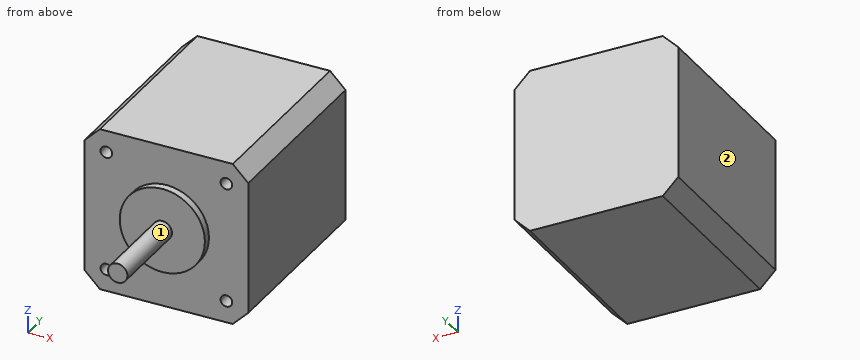
from build123d import *

# Parameters (mm, degrees)
F1_DEPTH = 48
F2_R     = 11
F3_DEPTH = 2
F4_R     = 2.5
F5_DEPTH = 22
F6_R     = 1.5
F7_DEPTH = 10


with BuildPart() as f1:
    # F0 (on Front) → F1 (new body)
    with BuildSketch(Plane.XZ):
        Polygon((17.15, 21.15), (0, 21.15), (-17.15, 21.15), (-21.15, 17.15), (-21.15, 0), (-21.15, -17.15), (-17.15, -21.15), (0, -21.15), (17.15, -21.15), (21.15, -17.15), (21.15, 0), (21.15, 17.15), align=None)
    extrude(amount=F1_DEPTH)

    # F2 (on face) → F3 (join)
    with BuildSketch(Plane.XZ.offset(48)):
        Circle(F2_R)
    extrude(amount=F3_DEPTH)

    # F4 (on face) → F5 (join)
    with BuildSketch(Plane.XZ.offset(50)):
        Circle(F4_R)
    extrude(amount=F5_DEPTH)

    # F6 (on face) → F7 (cut)
    with BuildSketch(Plane.XZ.offset(48)):
        with Locations((-15.5, 15.5)):
            Circle(F6_R)
        with Locations((15.5, 15.5)):
            Circle(F6_R)
        with Locations((-15.5, -15.5)):
            Circle(F6_R)
        with Locations((15.5, -15.5)):
            Circle(F6_R)
    extrude(amount=-F7_DEPTH, mode=Mode.SUBTRACT)


solid = f1.part
Geometry: final body of the model. Coordinates: model frame, mm. Face numbers are marked on the shaded views. A direction names the side the tool comes from. Give positions to 0.01 mm unless a question says otherwise; leave off trailing zeros. Write each loop counter-clockwise with the first axis right and the second up, starting at its lowest first coordinate (ties: lowest second). Pieces come first, ordered by that corner, then holes. Notation, with made-up numbers: M 26,30.5 L 85,30.5 A17 ccw 85,60.5 Z; hole C 73,23.5 d9. An arc over 180 degrees is marked long. Answer in a Markdown table with one row per item. Add a question column.
(1) Section C-C on z = 0. Return loops of the section in (x, y).
(2) Ray query, line 1 (Z direction, x = 15.5, y = -43.75); line 2 (Z direction, x = -15, y = -45); line 3 (Y direction, x = 0, z = 19.5). Return the intervals inside material, ascending.
(3) First-contact query: pin 1 (0.9 mm diameter, centred on x = 15, z = 15, fed in from -Y); pin 2 (4 mm diameter, centred on x = 15.5, z = 13, fed in from -Y); pin 3 (4 mm diameter, centred on x = 5.5, y = -52.5, fed in from +Z) (3 decimals). Flat tips, straight axial feed; report the tip coordinate or a pass-through.
(4) Section B-B on y = -17. Return loops of the section in (x, z), and give its area (3 significant figures).
(5) Section D-D on z = -6.5. Return loops of the section in (x, y).
(6) Reachability of the marked faces 1 and 2 from +Z, -Z, +X, -X, +Y, -Y: full face, straight path, thin tool, end or side. Return the list, or none.
(7) Section A-A on x = -15.5. Return loops of the section in (y, z).
Result set:
| question | item | result |
|---|---|---|
| 1 | outline | M -21.15,-48 L -11,-48 L -11,-50 L -2.5,-50 L -2.5,-72 L 2.5,-72 L 2.5,-50 L 11,-50 L 11,-48 L 21.15,-48 L 21.15,0 L -21.15,0 Z |
| 2 | line 1 | z = -21.15 to -17, -14 to 14, 17 to 21.15 |
| 2 | line 2 | z = -21.15 to -16.91, -14.09 to 14.09, 16.91 to 21.15 |
| 2 | line 3 | y = -48 to 0 |
| 3 | pin 1 | stops at y = -38 |
| 3 | pin 2 | stops at y = -48 |
| 3 | pin 3 | passes through |
| 4 | outline | M -21.15,-17.15 L -17.15,-21.15 L 17.15,-21.15 L 21.15,-17.15 L 21.15,17.15 L 17.15,21.15 L -17.15,21.15 L -21.15,17.15 Z |
| 4 | area | 1,760 mm^2 |
| 5 | outline | M -21.15,-48 L -8.87,-48 L -8.87,-50 L 8.87,-50 L 8.87,-48 L 21.15,-48 L 21.15,0 L -21.15,0 Z |
| 6 | face 1 | -Y |
| 6 | face 2 | +Z, -Z, -X, +Y, -Y |
| 7 | outline | M -48,-21.15 L 0,-21.15 L 0,21.15 L -48,21.15 L -48,17 L -38,17 L -38,14 L -48,14 L -48,-14 L -38,-14 L -38,-17 L -48,-17 Z |
